Part model, mm, in its own coordinate system. A direction names the side the tool comes from. Give positions to 0.01 mm unless a question says otherwise; leave off trailing zeros. Write each loop counter-clockwise with the first axis right and the second up, starting at its lowest first coordinate (ties: lowest second). Pieces come first, ordered by that corner, then holes. Notation, with made-up numbers: M 87,40.5 L 117,40.5 A14 ccw 117,60.5 Z; hole C -37,65.5 d3. An arc over 180 degrees is marked long. Use a Markdown table: item, result.
Autodesk Inventor part; units mm, degrees
ref_plane "YZ Plane" through (0, 0, 0) normal (1, 0, 0) x (0, 1, 0)
ref_plane "XZ Plane" through (0, 0, 0) normal (0, 1, 0) x (-1, 0, 0)
ref_plane "XY Plane" through (0, 0, 0) normal (0, 0, 1) x (1, 0, 0)
sketch "Sketch1" plane through (0, 0, 0) normal (0, 1, 0) x (-1, 0, 0)
  circle A0 centre (0, 0) radius 1.5
  circle A1 centre (0, 0) radius 2.5
  dimension "d0" = 3
  dimension "d1" = 5
extrude "Extrusion1" add sketch "Sketch1" along normal blind 12 contours A0
extrude "Extrusion2" add sketch "Sketch1" against normal blind 2.5 contours A0 | A1
thread "Thread1"
sketch "Sketch2" plane through (0, -2.5, 0) normal (0, -1, 0) x (1, 0, 0)
  line L0 (1.25, -0.7217) -> (0, -1.4434)
  line L1 (0, -1.4434) -> (-1.25, -0.7217)
  line L2 (-1.25, -0.7217) -> (-1.25, 0.7217)
  line L3 (-1.25, 0.7217) -> (0, 1.4434)
  line L4 (0, 1.4434) -> (1.25, 0.7217)
  line L5 (1.25, 0.7217) -> (1.25, -0.7217)
  point P0 (0, 0)
  point P1 (0, 0)
  point P2 (1.25, 0)
extrude "Extrusion3" cut sketch "Sketch2" against normal blind 2
properties part number "M4"
1. Drill centre lines: L1, parallel to Y at x = 1.2, z = -0.4; L2, parallel to Y at x = 1.75, z = 1; L3, parallel to Z at x = -1.05, y = -1.5. Where is each one in solid material? Low to high.
Findings below:
| item | result |
|---|---|
| L1 | -0.5 to 12 |
| L2 | -2.5 to 0 |
| L3 | -2.27 to -0.84, 0.84 to 2.27 |
2. Cut at D-D, the plane z = -2. Give the cut face in (x, y), then the cut area to 3 significant figures.
Findings below:
| item | result |
|---|---|
| outline | M -1.5,-2.5 L 1.5,-2.5 L 1.5,0 L -1.5,0 Z |
| area | 7.50 mm2 |
3. Drop flat-ended pins along their axis: P1, Ø1.6, axis at y = -1.5, z = 0.5, coming from the +X side; P2, Ø1, axis at x = -1, y = 8, coming from the +Z side. Give the stop position or say it passes through.
Findings below:
| item | result |
|---|---|
| P1 | x = 2.5 |
| P2 | z = 1.41 |
4. Cut at A-A, the plane z = 0. Give the cut face in (x, y), then the cut area to 3 significant figures.
Findings below:
| item | result |
|---|---|
| outline | M -2.5,-2.5 L -1.25,-2.5 L -1.25,-0.5 L 1.25,-0.5 L 1.25,-2.5 L 2.5,-2.5 L 2.5,0 L 1.5,0 L 1.5,12 L -1.5,12 L -1.5,0 L -2.5,0 Z |
| area | 43.5 mm2 |
5. Tool access for faces 1 (the flat face through (0, 12, 0)), 2 (the cylindrical face through (1.5, 5.92, -0.07)), 3 (the flat face through (1.25, -2, 0)): list every direction of +Z, -Z, +X, -X, +Y, -Y with a clear straight run to the whole face (end or side of a thin tool).
Findings below:
| item | result |
|---|---|
| face 1 | +Z, -Z, +X, -X, +Y |
| face 2 | +Y |
| face 3 | -Y |
6. Cut at C-C, the plane x = 0.75. Give the cut face in (y, z).
Findings below:
| item | result |
|---|---|
| outline | M -2.5,-2.38 L 0,-2.38 L 0,-1.3 L 12,-1.3 L 12,1.3 L 0,1.3 L 0,2.38 L -2.5,2.38 L -2.5,1.01 L -0.5,1.01 L -0.5,-1.01 L -2.5,-1.01 Z |
7. Cut at B-B, the plane y = 6. Give the cut face in (x, z), then the cut area to 3 significant figures.
Findings below:
| item | result |
|---|---|
| outline | C 0,0 d3 |
| area | 7.07 mm2 |
8. Two-plate mould, pull along Z, no slides. Class faces 4 (the flat face through (-2, 0, 0)), 5 (the cylindrical face through (0.54, -1.23, -2.44)), 6 (the flat face through (-0.616, -1.514, -1.088)): released by +Z, released by -Z, zero draft, split by the parting line, or undercut.
Findings below:
| item | result |
|---|---|
| face 4 | zero draft |
| face 5 | split by the parting line |
| face 6 | undercut |
